from build123d import *

# Parameters (mm, degrees)
SKETCH1_W           = 558.8
SKETCH1_H           = 38.1
BOSS_EXTRUDE1_DEPTH = 3.175
SKETCH2_W           = 558.8
SKETCH2_H           = 3.175
BOSS_EXTRUDE2_DEPTH = 44.45
FILLET1_R           = 2.54
SKETCH3_R           = 3.175
CUT_EXTRUDE1_DEPTH  = 44.45
CUT_EXTRUDE2_DEPTH  = 650.113
BOSS_EXTRUDE3_DEPTH = 558.8
SKETCH6_W           = 32.897959938
SKETCH6_H           = 44.45
CUT_EXTRUDE3_DEPTH  = 558.8
FILLET2_R           = 2.54


with BuildPart() as part:
    # Sketch1 → Boss-Extrude1 (new body)
    with BuildSketch(Plane.XY):
        with Locations((279.4, 19.05)):
            Rectangle(SKETCH1_W, SKETCH1_H)
    extrude(amount=BOSS_EXTRUDE1_DEPTH)

    # Sketch2 → Boss-Extrude2 (add)
    with BuildSketch(Plane.XY.offset(3.175)):
        with Locations((279.4, 36.5125)):
            Rectangle(SKETCH2_W, SKETCH2_H)
        with Locations((279.4, 1.5875)):
            Rectangle(SKETCH2_W, SKETCH2_H)
    extrude(amount=BOSS_EXTRUDE2_DEPTH)

    # Fillet1
    fillet1_edges = [part.edges().sort_by_distance(p)[0] for p in [
        (279.4, 34.925, 3.175),
        (279.4, 3.175, 3.175),
        (279.4, 0, 0),
        (279.4, 38.1, 0),
    ]]
    fillet(fillet1_edges, radius=FILLET1_R)

    # Sketch3 → Cut-Extrude1 (cut)
    with BuildSketch(Plane(origin=(0, 38.1, 0), x_dir=(1, 0, 0), z_dir=(0, 1, 0))):
        with Locations((12.7, -35.1028)):
            Circle(SKETCH3_R)
        with Locations((38.1, -35.1028)):
            Circle(SKETCH3_R)
        with Locations((63.5, -35.1028)):
            Circle(SKETCH3_R)
        with Locations((88.9, -35.1028)):
            Circle(SKETCH3_R)
        with Locations((114.3, -35.1028)):
            Circle(SKETCH3_R)
        with Locations((139.7, -35.1028)):
            Circle(SKETCH3_R)
        with Locations((165.1, -35.1028)):
            Circle(SKETCH3_R)
        with Locations((190.5, -35.1028)):
            Circle(SKETCH3_R)
        with Locations((215.9, -35.1028)):
            Circle(SKETCH3_R)
        with Locations((241.3, -35.1028)):
            Circle(SKETCH3_R)
        with Locations((266.7, -35.1028)):
            Circle(SKETCH3_R)
        with Locations((292.1, -35.1028)):
            Circle(SKETCH3_R)
        with Locations((317.5, -35.1028)):
            Circle(SKETCH3_R)
        with Locations((342.9, -35.1028)):
            Circle(SKETCH3_R)
        with Locations((368.3, -35.1028)):
            Circle(SKETCH3_R)
        with Locations((393.7, -35.1028)):
            Circle(SKETCH3_R)
        with Locations((419.1, -35.1028)):
            Circle(SKETCH3_R)
        with Locations((444.5, -35.1028)):
            Circle(SKETCH3_R)
        with Locations((469.9, -35.1028)):
            Circle(SKETCH3_R)
        with Locations((495.3, -35.1028)):
            Circle(SKETCH3_R)
        with Locations((520.7, -35.1028)):
            Circle(SKETCH3_R)
        with Locations((546.1, -35.1028)):
            Circle(SKETCH3_R)
        with Locations((38.1, -9.7028)):
            Circle(SKETCH3_R)
        with Locations((63.5, -9.7028)):
            Circle(SKETCH3_R)
        with Locations((88.9, -9.7028)):
            Circle(SKETCH3_R)
        with Locations((114.3, -9.7028)):
            Circle(SKETCH3_R)
        with Locations((139.7, -9.7028)):
            Circle(SKETCH3_R)
        with Locations((165.1, -9.7028)):
            Circle(SKETCH3_R)
        with Locations((190.5, -9.7028)):
            Circle(SKETCH3_R)
        with Locations((215.9, -9.7028)):
            Circle(SKETCH3_R)
        with Locations((241.3, -9.7028)):
            Circle(SKETCH3_R)
        with Locations((266.7, -9.7028)):
            Circle(SKETCH3_R)
        with Locations((292.1, -9.7028)):
            Circle(SKETCH3_R)
        with Locations((317.5, -9.7028)):
            Circle(SKETCH3_R)
        with Locations((342.9, -9.7028)):
            Circle(SKETCH3_R)
        with Locations((368.3, -9.7028)):
            Circle(SKETCH3_R)
        with Locations((393.7, -9.7028)):
            Circle(SKETCH3_R)
        with Locations((419.1, -9.7028)):
            Circle(SKETCH3_R)
        with Locations((444.5, -9.7028)):
            Circle(SKETCH3_R)
        with Locations((469.9, -9.7028)):
            Circle(SKETCH3_R)
        with Locations((495.3, -9.7028)):
            Circle(SKETCH3_R)
        with Locations((520.7, -9.7028)):
            Circle(SKETCH3_R)
        with Locations((546.1, -9.7028)):
            Circle(SKETCH3_R)
        with Locations((12.7, -9.7028)):
            Circle(SKETCH3_R)
    extrude(amount=-CUT_EXTRUDE1_DEPTH, mode=Mode.SUBTRACT)

    # Sketch4 → Cut-Extrude2 (cut)
    with BuildSketch(Plane(origin=(558.8, 0, 0), x_dir=(0, 0, -1), z_dir=(1, 0, 0))):
        Polygon((-2.54, 25.4), (13.885485297, 25.4), (13.885485297, 51.082453825), (-54.332543736, 51.082453825), (-54.332543736, 25.4), align=None)
    extrude(amount=-CUT_EXTRUDE2_DEPTH, mode=Mode.SUBTRACT)

    # Mirror1: part across plane


with BuildPart() as part_1:
    add(part.part)
    add(part.part.mirror(Plane(origin=(-91.313, 25.4, 2.54), x_dir=(0, 0, 1), z_dir=(0, -1, 0))))

    # Sketch5 → Boss-Extrude3 (add)
    with BuildSketch(Plane(origin=(558.8, 0, 0), x_dir=(0, 0, -1), z_dir=(1, 0, 0))):
        with BuildLine():
            Line((3.175, 50.8), (-2.54, 50.8))
            ThreePointArc((-2.54, 50.8), (-0.743948776, 50.056051224), (0, 48.26))
            Line((0, 48.26), (0, 47.625))
            Line((0, 47.625), (3.175, 47.625))
            Line((3.175, 47.625), (3.175, 50.8))
        make_face()
        with BuildLine():
            Line((-2.54, 50.8), (-3.966383497, 50.8))
            Line((-3.966383497, 50.8), (-3.966383497, 47.625))
            Line((-3.966383497, 47.625), (0, 47.625))
            Line((0, 47.625), (0, 48.26))
            ThreePointArc((0, 48.26), (-0.743948776, 50.056051224), (-2.54, 50.8))
        make_face()
        Polygon((6.35, 50.8), (3.175, 50.8), (3.175, 47.625), (3.175, 3.175), (3.175, 0), (6.35, 0), align=None)
        with BuildLine():
            ThreePointArc((0, 2.54), (-0.743948776, 0.743948776), (-2.54, 0))
            Line((-2.54, 0), (3.175, 0))
            Line((3.175, 0), (3.175, 3.175))
            Line((3.175, 3.175), (0, 3.175))
            Line((0, 3.175), (0, 2.54))
        make_face()
        with BuildLine():
            Line((-5.715, 3.175), (-5.715, 0))
            Line((-5.715, 0), (-2.54, 0))
            ThreePointArc((-2.54, 0), (-0.743948776, 0.743948776), (0, 2.54))
            Line((0, 2.54), (0, 3.175))
            Line((0, 3.175), (-5.715, 3.175))
        make_face()
    extrude(amount=-BOSS_EXTRUDE3_DEPTH)

    # Sketch6 → Cut-Extrude3 (cut)
    with BuildSketch(Plane(origin=(558.8, 0, 0), x_dir=(0, 0, -1), z_dir=(1, 0, 0))):
        with Locations((-13.273979969, 25.4)):
            Rectangle(SKETCH6_W, SKETCH6_H)
    extrude(amount=-CUT_EXTRUDE3_DEPTH, mode=Mode.SUBTRACT)

    # Fillet2
    fillet2_edges = [part_1.edges().sort_by_distance(p)[0] for p in [
        (279.4, 0, -6.35),
        (279.4, 3.175, -3.175),
        (279.4, 47.625, -3.175),
        (279.4, 50.8, -6.35),
    ]]
    fillet(fillet2_edges, radius=FILLET2_R)


solid = part_1.part
Could you check a few things on this model? Use its own coordinates, in mm. A direction names the side the tool comes from. Give positions to 0.01 mm unless a question says otherwise; leave off trailing zeros. Order: outer loops, then holes, each group sorted by start corner. A loop starts at its lowest first (then second) coordinate and runs counter-clockwise, first axis right, second up. Notation, with made-up numbers: (38.25, 16) - (62.25, 16) arc R33 ccw to (62.25, 50) - close; hole circle Ø2 at (-7.75, -2.75). An arc over 180 degrees is marked (long way). Return JSON: item names as keys, results as strings. Group by question number.
Q1. Suppose I cut it at B-B, the plane y = 39. Please give me the cut outline in (x, z) (3 decimals), and give its area (3 significant figures).
Q2. Which directions (+Z, -Z, +X, -X, +Y, -Y) give clear straight access to the entire face, cutting with the end or side of a thin tool? Please do faces 1 (the face through (275, 3.175, 23)), 2 (the face through (275, 50.8, 22)).
Q3. Thinking about a two-plate mould opening in Y: for faces 3 (the face through (283, 47.625, 24)), 4 (the face through (283, 0, 22)), 5 (the face through (283, 25, -6.35)), which applies, pulls with the +Y half, pulls with the -Y half, needs draft (parallel to the pull), parting line crosses it, or undercut?
Q4. Suppose I cut it at A-A, the plane z = 27. Please give me the cut outline in (x, y) (3 decimals).
Q5. Please list where these lines run through material, in increasing order: line 1 along Z through (x, y) = (241, 48) (3 decimals); line 2 along Y through (x, z) = (260.5, 41.5) (3 decimals); line 3 along Z through (x, y) = (469.9, 49.35) (3 decimals). Write a range as [from, to].
Q6. Will these pins go through, and if not, where does the flat tip stop? pin 1 Ø6 at (x, y) = (257.5, 6.5) entering from +Z; pin 2 Ø5 at (x, y) = (183, 20.5) entering from +Z (3 decimals).
Resolved:
{
 "1": {"outline": "(0, -6.35) - (558.8, -6.35) - (558.8, -3.175) - (0, -3.175) - close", "area": "1,770 mm2"},
 "2": {"face 1": "+Z, +X, -X", "face 2": "+Z, -Z, +X, -X, +Y"},
 "3": {"face 3": "undercut", "face 4": "pulls with the -Y half", "face 5": "needs draft"},
 "4": {"outline": "(0, 0) - (558.8, 0) - (558.8, 3.175) - (0, 3.175) - close; (0, 47.625) - (558.8, 47.625) - (558.8, 50.8) - (0, 50.8) - close"},
 "5": {"line 1": "z = [-6.35, 6.542], [12.864, 31.942], [38.264, 47.625]", "line 2": "y = [0, 3.175], [47.625, 50.8]", "line 3": "z = [-6.104, 6.528], [12.878, 31.928], [38.278, 47.625]"},
 "6": {"pin 1": "stops at z = -1.88", "pin 2": "stops at z = -3.175"}
}
